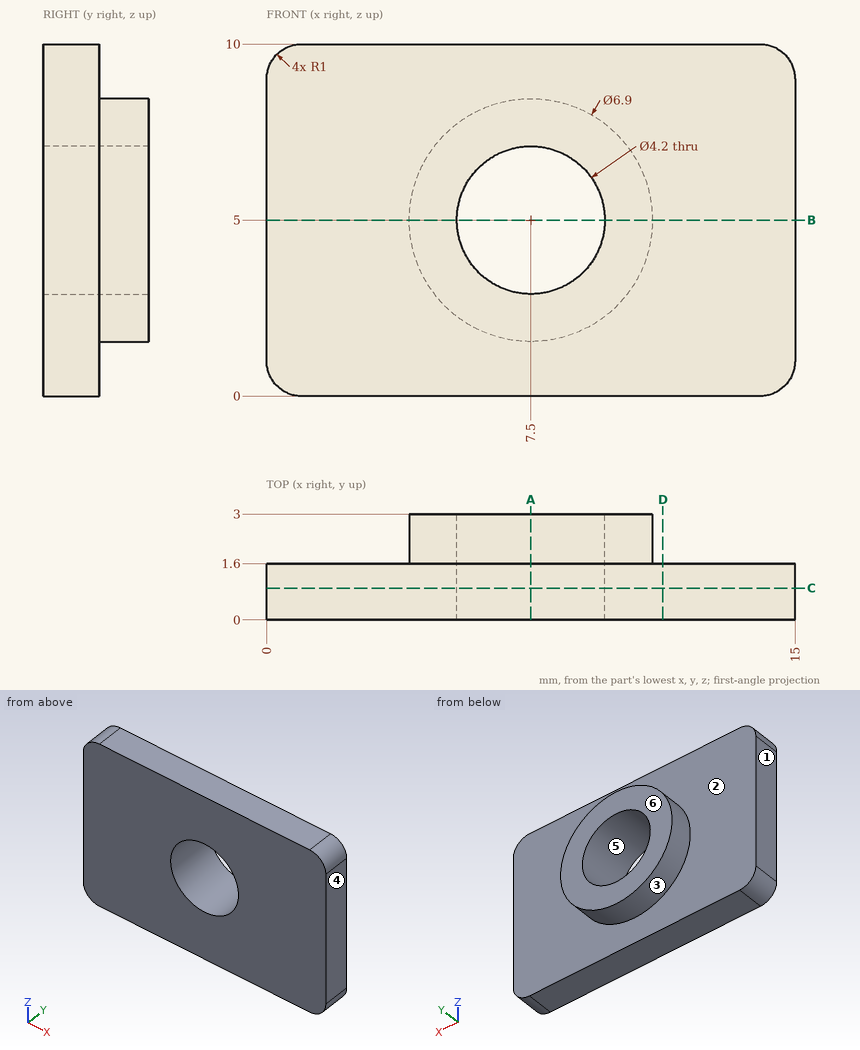
Print and shaded views of the part. All mm, measured from the part's lowest x, y and z. A direction names the side the tool comes from. Coordinates: 2 decimals unless noted, no trailing zeros. Loops run counter-clockwise (first coordinate to the right, second up) from the corner with the lowest first, then second, coordinate; pieces in that order, holes last. Notation, with made-up numbers: (-1, 19) - (50, 19) arc R26 ccw to (50, 36) - close; hole circle Ø8 at (50.25, -36). An arc over 180 degrees is marked (long way). Use one line per item in the form item = value. Start each with the question number.
1) Band-saw the part on A-A (x = 7.5). Give the cut face in (y, z), and give its area (3 significant figures).
2) Band-saw the part on D-D (x = 11.25). Give the cut face in (y, z).
3) Flat gauge pin, fed straight in: pin 1 (5 mm diameter, centred on x = 8, z = 3.5, fed in from +Y). Where does the tip first touch, or does it go through?
4) Two-plate mould, pull along X, no slides. Class the marked faces 3, 4, 5 and 6: +X half, -X half, draft (parallel to the pull), parting line (faces both ways), or undercut.
5) Band-saw the part on B-B (z = 5). Give the cut face in (x, y), and give its area (3 significant figures).
6) Tool access for the marked faces 1 and 2: list every direction of +Z, -Z, +X, -X, +Y, -Y with a clear straight run to the whole face (end or side of a thin tool).
7) Drill centre lines: L1, parallel to X at y = 0.9, z = 5; L2, parallel to X at y = 1.7, z = 5; L3, parallel to Y at x = 11.75, z = 2. Where is each one in solid material? Low to high. Write a range as from..to.
8) Band-saw the part on C-C (y = 0.9). Give the cut face in (x, z).
Check values:
q1.outline = (0, 0) - (1.6, 0) - (1.6, 1.55) - (3, 1.55) - (3, 2.9) - (0, 2.9) - close; (0, 7.1) - (3, 7.1) - (3, 8.45) - (1.6, 8.45) - (1.6, 10) - (0, 10) - close
q1.area = 13.1 mm2
q2.outline = (0, 0) - (1.6, 0) - (1.6, 10) - (0, 10) - close
q3.pin_1 = 3
q4.face_3 = parting line
q4.face_4 = +X half
q4.face_5 = undercut
q4.face_6 = draft
q5.outline = (0, 0) - (5.4, 0) - (5.4, 3) - (4.05, 3) - (4.05, 1.6) - (0, 1.6) - close; (9.6, 0) - (15, 0) - (15, 1.6) - (10.95, 1.6) - (10.95, 3) - (9.6, 3) - close
q5.area = 21.1 mm2
q6.face_1 = +Z, -Z, -X, +Y, -Y
q6.face_2 = +Y
q7.L1 = 0..5.4, 9.6..15
q7.L2 = 4.05..5.4, 9.6..10.95
q7.L3 = 0..1.6
q8.outline = (0, 1) arc R1 ccw to (1, 0) - (14, 0) arc R1 ccw to (15, 1) - (15, 9) arc R1 ccw to (14, 10) - (1, 10) arc R1 ccw to (0, 9) - close; hole circle Ø4.2 at (7.5, 5)
